from build123d import *

# Parameters (mm, degrees)
CROQUIS1_W              = 14
CROQUIS1_H              = 6
SALIENTE_EXTRUIR1_DEPTH = 40
SALIENTE_EXTRUIR4_DEPTH = 25
CORTAR_EXTRUIR1_REACH   = 59.411
CROQUIS3_R              = 3


with BuildPart() as part:
    # Croquis1 → Saliente-Extruir1 (new body)
    with BuildSketch(Plane(origin=(0, 0, 0), x_dir=(1, 0, 0), z_dir=(0, 1, 0))):
        Polygon((-11, 8), (-9, 10), (9, 10), (11, 8), (11, -8), (9, -10), (-9, -10), (-11, -8), align=None)
        Rectangle(CROQUIS1_W, CROQUIS1_H, mode=Mode.SUBTRACT)
    extrude(amount=SALIENTE_EXTRUIR1_DEPTH)

    # Croquis2 → Saliente-Extruir4 (add)
    with BuildSketch(Plane(origin=(11, 0, 0), x_dir=(0, 0, -1), z_dir=(1, 0, 0))):
        with BuildLine():
            Line((-3.505117141, 9.641441068), (-5.99727833, 17.243357445))
            ThreePointArc((-5.99727833, 17.243357445), (-5.88119691, 18.769683379), (-4.719839533, 19.766876837))
            Line((-4.719839533, 19.766876837), (0.98159775, 21.635997729))
            ThreePointArc((0.98159775, 21.635997729), (2.507923683, 21.519916309), (3.505117141, 20.358558932))
            Line((3.505117141, 20.358558932), (5.99727833, 12.756642555))
            ThreePointArc((5.99727833, 12.756642555), (5.88119691, 11.230316621), (4.719839533, 10.233123163))
            Line((4.719839533, 10.233123163), (-0.98159775, 8.364002271))
            ThreePointArc((-0.98159775, 8.364002271), (-2.507923683, 8.480083691), (-3.505117141, 9.641441068))
        make_face()
    extrude(amount=SALIENTE_EXTRUIR4_DEPTH)

    # Croquis3 → Cortar-Extruir1 (cut, up to next)
    with BuildSketch(Plane.XY.offset(10), mode=Mode.PRIVATE) as cortar_extruir1_sk1:
        with Locations((0, 10)):
            Circle(CROQUIS3_R)
    cortar_extruir1_tool1 = extrude(cortar_extruir1_sk1.sketch, amount=-CORTAR_EXTRUIR1_REACH, mode=Mode.PRIVATE) & part.part
    # Croquis3 → Cortar-Extruir1 (cut, up to next)
    with BuildSketch(Plane.XY.offset(10), mode=Mode.PRIVATE) as cortar_extruir1_sk2:
        with Locations((0, 25)):
            Circle(CROQUIS3_R)
    cortar_extruir1_tool2 = extrude(cortar_extruir1_sk2.sketch, amount=-CORTAR_EXTRUIR1_REACH, mode=Mode.PRIVATE) & part.part
    add(cortar_extruir1_tool1.solids().sort_by_distance((0, 10, 10))[0], mode=Mode.SUBTRACT)
    add(cortar_extruir1_tool2.solids().sort_by_distance((0, 25, 10))[0], mode=Mode.SUBTRACT)


solid = part.part
Work out the finished part from the listing and answer in its coordinate system (mm). A direction names the side the tool comes from. Round coordinates to 2 decimals unless told otherwise and drop trailing zeros. Loops run counter-clockwise (first coordinate to the right, second up) from the corner with the lowest first, then second, coordinate; pieces in that order, holes last. Notation, with made-up numbers: (5.5, 13) - (49.5, 13) arc R24 cw to (49.5, 48) - close; hole circle Ø4 at (64, 17). An arc over 180 degrees is marked (long way). Use one line per item in the form item = value. Start each with the question number.
(1) Find section B-B on y = 6. Determine the outline of the cut face in (x, z).
(2) Find section A-A on x = 0. Determine the outline of the cut face in (y, z).
(3) Find section D-D on x = 14.5. Determine the outline of the cut face in (y, z).
(4) Determine the mould class of faces 1 (the face through (-3, 10, 7)), 2 (the face through (10, 20, 9)), 3 (the face through (7, 20, 0)) for opening direction Z: +Z half, -Z half, draft (parallel to the pull), parting line (faces both ways), or undercut.
(5) Which of the six approach directions +Z, -Z, +X, -X, +Y, -Y give full straight-line access (tool end or side, diameter ignored) to faces 4 (the face through (23.32, 21.53, -2.49)), 5 (the face through (-7, 20, 0)), 6 (the face through (-0.65, 22.07, 6.55))?
(6) Consider line 1 (Y direction, x = 0, z = 5.5); line 2 (Z direction, x = -5.5, y = 37.5); line 3 (Y direction, x = 1, z = 6). Determine where each line is inside the solid, lowest interval first.
(7) Find section C-C on y = 25. Determine the outline of the cut face in (x, z).
(8) Flat-ended cylindrical pins translate along their axes: P1, Ø6, axis at x = 29, z = 4, coming from the +Y side; P2, Ø1, axis at x = 31, z = -3.5, coming from the -Y side; P3, Ø1, axis at y = 6.5, z = -7.5, coming from the +X side; P4, Ø3, axis at y = 22, z = -0.5, coming from the +X side. Find the tip coordinate at first contact, or state that the pin passes through.
Answer list:
q1.outline = (-11, -8) - (-9, -10) - (9, -10) - (11, -8) - (11, 8) - (9, 10) - (-9, 10) - (-11, 8) - close; hole (-7, -3) - (7, -3) - (7, 3) - (-7, 3) - close
q2.outline = (0, -10) - (40, -10) - (40, -3) - (0, -3) - close; (0, 3) - (7, 3) - (7, 10) - (0, 10) - close; (13, 3) - (22, 3) - (22, 10) - (13, 10) - close; (28, 3) - (40, 3) - (40, 10) - (28, 10) - close
q3.outline = (8.36, 0.98) - (10.23, -4.72) arc R2 ccw to (12.76, -6) - (20.36, -3.51) arc R2 ccw to (21.64, -0.98) - (19.77, 4.72) arc R2 ccw to (17.24, 6) - (9.64, 3.51) arc R2 ccw to start
q4.face_1 = draft
q4.face_2 = +Z half
q4.face_3 = undercut
q5.face_4 = +X, +Y
q5.face_5 = +Y, -Y
q5.face_6 = +Z
q6.line_1 = 0 to 7, 13 to 22, 28 to 40
q6.line_2 = -10 to -3, 3 to 10
q6.line_3 = 0 to 7.17, 12.83 to 22.17, 27.83 to 40
q7.outline = (-11, -8) - (-9, -10) - (9, -10) - (11, -8) - (11, 8) - (9, 10) - (3, 10) - (3, 3) - (7, 3) - (7, -3) - (-7, -3) - (-7, 3) - (-3, 3) - (-3, 10) - (-9, 10) - (-11, 8) - close
q8.P1 = 20.99
q8.P2 = 9.67
q8.P3 = 11
q8.P4 = 36
